Can you work these out from the model? Positions are in its coordinate system, mm. A direction names the side the tool comes from. Round coordinates to 2 decimals unless told otherwise and drop trailing zeros. Loops run counter-clockwise (first coordinate to the right, second up) from the corner with the lowest first, then second, coordinate; pieces in that order, holes last. Notation, with made-up numbers: (82, -18.5) -> (137, -18.5) arc R18 cw to (137, -4.5) -> close; hole circle Ø7 at (64, 70). An arc over 180 degrees is marked (long way). Answer as a JSON object with one key per item and string values.
```python
from build123d import *

# Parameters (mm, degrees)
F1_DEPTH = 25.4
F2_R     = 2.54


with BuildPart() as f1:
    # F0 (on Top) → F1 (new body)
    with BuildSketch(Plane.XY):
        Polygon((50.462863, 51.598176), (-38.437137, 51.598176), (-38.437137, 38.898176), (37.762863, 38.898176), (37.762863, 19.848176), (-38.437137, 19.848176), (-38.437137, -37.301824), (37.762863, -37.301824), (37.762863, -17.442089), (25.062863, -17.442089), (25.062863, -24.601824), (-25.737137, -24.601824), (-25.737137, 7.148176), (50.462863, 7.148176), align=None)
    extrude(amount=F1_DEPTH)

    # F2
    f2_edges = [f1.edges().sort_by_distance(p)[0] for p in [
        (-38.437137, 51.598176, 12.7),
        (50.462863, 51.598176, 12.7),
        (50.462863, 7.148176, 12.7),
        (-38.437137, 19.848176, 12.7),
        (-38.437137, -37.301824, 12.7),
        (37.762863, -37.301824, 12.7),
        (25.062863, -17.442089, 12.7),
        (37.762863, -17.442089, 12.7),
        (-25.737137, 7.148176, 12.7),
        (-25.737137, -24.601824, 12.7),
        (25.062863, -24.601824, 12.7),
        (-38.437137, 38.898176, 12.7),
        (-38.437137, -8.726824, 25.4),
        (-0.337137, -37.301824, 25.4),
        (37.762863, -27.371956, 25.4),
        (31.412863, -17.442089, 25.4),
        (25.062863, -21.021956, 25.4),
        (-0.337137, -24.601824, 25.4),
        (-25.737137, -8.726824, 25.4),
        (12.362863, 7.148176, 25.4),
        (50.462863, 29.373176, 25.4),
        (6.012863, 51.598176, 25.4),
        (-38.437137, 45.248176, 25.4),
        (-0.337137, 38.898176, 25.4),
        (37.762863, 29.373176, 25.4),
        (-0.337137, 19.848176, 25.4),
        (-38.437137, -8.726824, 0),
        (-0.337137, -37.301824, 0),
        (37.762863, -27.371956, 0),
        (31.412863, -17.442089, 0),
        (25.062863, -21.021956, 0),
        (-0.337137, -24.601824, 0),
        (-25.737137, -8.726824, 0),
        (12.362863, 7.148176, 0),
        (50.462863, 29.373176, 0),
        (6.012863, 51.598176, 0),
        (-38.437137, 45.248176, 0),
        (-0.337137, 38.898176, 0),
        (37.762863, 29.373176, 0),
        (-0.337137, 19.848176, 0),
    ]]
    fillet(f2_edges, radius=F2_R)


solid = f1.part
```
Q1. I'm going to push flat-ended pins straight in: pin 1 (6 mm diameter, centred on x = 32, y = -19.5, fed in from +Z); pin 2 (3 mm diameter, centred on x = -19.5, y = -23.5, fed in from -Z); pin 3 (12 mm diameter, centred on x = 24.5, y = -11.5, fed in from +Z). Where does each tip first touch, or does it pass through?
Determined:
{"pin 1": "z = 25.4", "pin 2": "z = 1.17", "pin 3": "through"}
Q2. If I drill on L1, parallel to Y at x = 15.5, z = 20.75; L2, parallel to Y at x = 28, z = 21.5; L3, parallel to Y at x = -31, z = 10.75, over which ranges is the centre line in solid material (lowest first)? Write a range as [from, to].
Determined:
{"L1": "[-37.3, -24.6], [7.15, 19.85], [38.9, 51.6]", "L2": "[-37.3, -17.44], [7.15, 19.85], [38.9, 51.6]", "L3": "[-37.3, 19.85], [38.9, 51.6]"}
Q3. I want a section at D-D, the plane y = -18.5. Write out the boundary of the cut face in (x, z), then the cut area to 3 significant figures.
Determined:
{"outline": "(-38.44, 2.54) arc R2.54 ccw to (-35.9, 0) -> (-28.28, 0) arc R2.54 ccw to (-25.74, 2.54) -> (-25.74, 22.86) arc R2.54 ccw to (-28.28, 25.4) -> (-35.9, 25.4) arc R2.54 ccw to (-38.44, 22.86) -> close; (25.54, 2.54) arc R2.06 ccw to (27.6, 0.48) -> (35.22, 0.48) arc R2.06 ccw to (37.29, 2.54) -> (37.29, 22.86) arc R2.06 ccw to (35.22, 24.92) -> (27.6, 24.92) arc R2.06 ccw to (25.54, 22.86) -> close", "area": "601 mm²"}
Q4. I want a section at A-A, the plane x = 9. Write out the boundary of the cut face in (y, z).
Determined:
{"outline": "(-37.3, 2.54) arc R2.54 ccw to (-34.76, 0) -> (-27.14, 0) arc R2.54 ccw to (-24.6, 2.54) -> (-24.6, 22.86) arc R2.54 ccw to (-27.14, 25.4) -> (-34.76, 25.4) arc R2.54 ccw to (-37.3, 22.86) -> close; (7.15, 2.54) arc R2.54 ccw to (9.69, 0) -> (17.31, 0) arc R2.54 ccw to (19.85, 2.54) -> (19.85, 22.86) arc R2.54 ccw to (17.31, 25.4) -> (9.69, 25.4) arc R2.54 ccw to (7.15, 22.86) -> close; (38.9, 2.54) arc R2.54 ccw to (41.44, 0) -> (49.06, 0) arc R2.54 ccw to (51.6, 2.54) -> (51.6, 22.86) arc R2.54 ccw to (49.06, 25.4) -> (41.44, 25.4) arc R2.54 ccw to (38.9, 22.86) -> close"}
Q5. We'd pull the mould along Y, two halves only. Please class faces 4 (the cylindrical face through (25.827, -18.166, 12.842)), 5 (the cylindrical face through (37.039, -27.268, 0.764)), 6 (the cylindrical face through (0.161, -36.578, 24.636)): pulls with the +Y half, pulls with the -Y half, needs draft (parallel to the pull), parting line crosses it, or undercut.
Determined:
{"face 4": "undercut", "face 5": "needs draft", "face 6": "pulls with the -Y half"}
Q6. On a 3-axis mill with a long thin cutter (end or side, diameter ignored), from which of +Z, -Z, +X, -X, +Y, -Y can I reach the whole of each face in a straight line? I mean faces 1 (the flat face through (0, -24.602, 13)), 2 (the flat face through (37.763, 30, 13)), 3 (the cylindrical face through (-0.66, -25.33, 0.76)). Say none if no direction works.
Determined:
{"face 1": "+Z, -Z", "face 2": "+Z, -Z, -X", "face 3": "-Z"}
Q7. I want a section at B-B, the plane y = -4. Write out the boundary of the cut face in (x, z).
Determined:
{"outline": "(-38.44, 2.54) arc R2.54 ccw to (-35.9, 0) -> (-28.28, 0) arc R2.54 ccw to (-25.74, 2.54) -> (-25.74, 22.86) arc R2.54 ccw to (-28.28, 25.4) -> (-35.9, 25.4) arc R2.54 ccw to (-38.44, 22.86) -> close"}
Q8. I want a section at C-C, the plane z = 5.25. Write out the boundary of the cut face in (x, y), then the cut area to 3 significant figures.
Determined:
{"outline": "(-38.44, -34.76) arc R2.54 ccw to (-35.9, -37.3) -> (35.22, -37.3) arc R2.54 ccw to (37.76, -34.76) -> (37.76, -19.98) arc R2.54 ccw to (35.22, -17.44) -> (27.6, -17.44) arc R2.54 ccw to (25.06, -19.98) -> (25.06, -22.06) arc R2.54 cw to (22.52, -24.6) -> (-23.2, -24.6) arc R2.54 cw to (-25.74, -22.06) -> (-25.74, 4.61) arc R2.54 cw to (-23.2, 7.15) -> (47.92, 7.15) arc R2.54 ccw to (50.46, 9.69) -> (50.46, 49.06) arc R2.54 ccw to (47.92, 51.6) -> (-35.9, 51.6) arc R2.54 ccw to (-38.44, 49.06) -> (-38.44, 41.44) arc R2.54 ccw to (-35.9, 38.9) -> (37.76, 38.9) -> (37.76, 19.85) -> (-35.9, 19.85) arc R2.54 ccw to (-38.44, 17.31) -> close", "area": "3,950 mm²"}
